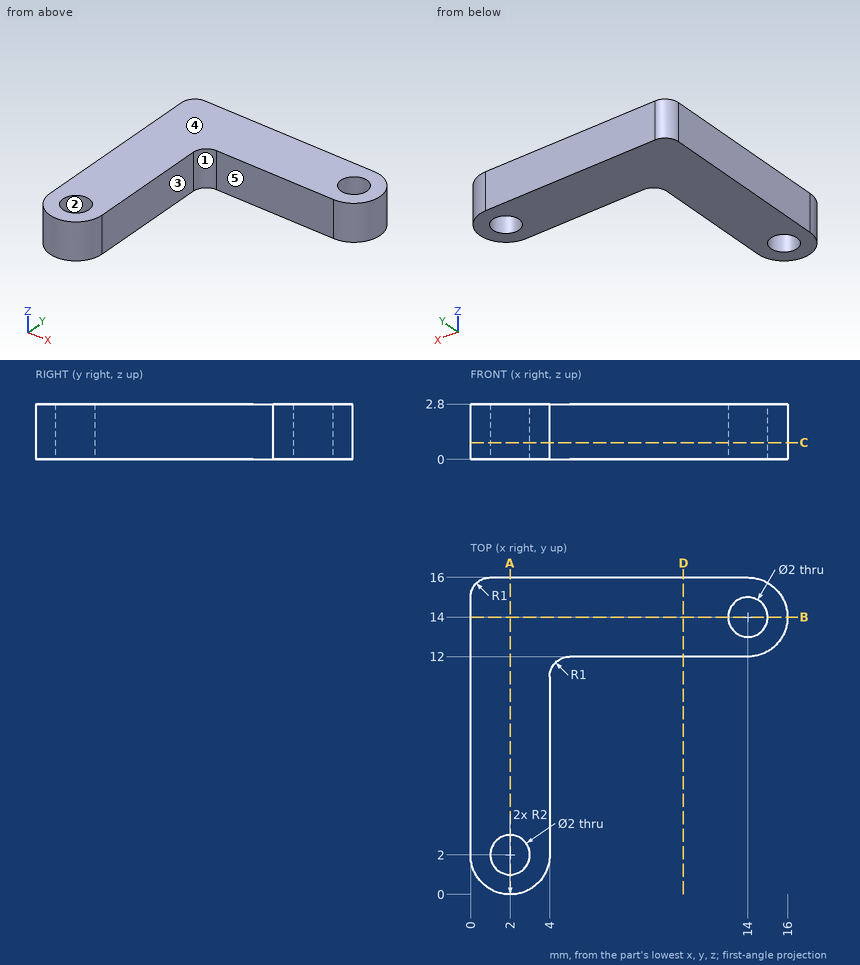
Part print with two shaded views. Sizes in mm from the minimum x, y, z corner. A direction names the side the tool comes from. Round coordinates to 2 decimals unless told otherwise and drop trailing zeros. Order: outer loops, then holes, each group sorted by start corner. A loop starts at its lowest first (then second) coordinate and runs counter-clockwise, first axis right, second up.
(1) 3-axis set-ups, long thin cutter, end or side, ignore diameter. For the marked faces 4 and 5: which of +Z, -Z, +X, -X, +Y, -Y reach the whole face in a straight line?
(2) Band-saw the part on A-A (x = 2). List the corners of the cut face in (y, z), then the cut area to 3 significant figures.
(3) Band-saw the part on C-C (z = 0.85). List the corners of the cut face in (x, y).
(4) Band-saw the part on D-D (x = 10.75). List the corners of the cut face in (y, z).
(5) Pull direction Y, two halves, no side cores. Call the marked faces 1, 2 and 3: released by +Y, released by -Y, zero draft, split by the parting line, or undercut.
(6) Band-saw the part on B-B (y = 14). List the corners of the cut face in (x, z), then the cut area to 3 significant figures.
(7) Pin check, flat tips, straight feed: pin 1 (6 mm diameter, centred on x = 5.5, y = 10, fed in from +Z); pin 2 (1.4 mm diameter, centred on y = 6, z = 1, fed in from +X). Stop position of each tip, or through.
(8) Drill centre lines: line 1 (Y direction, x = 14, z = 2); line 2 (Y direction, x = 6, z = 0.6); line 3 (X direction, y = 7.5, z = 0.1). Where is each one in solid material? Low to high.
Verdict:
1. face 4: +Z, +X, -X, +Y, -Y
1. face 5: +Z, -Z, +X, -Y
2. outline: (0, 0) - (1, 0) - (1, 2.8) - (0, 2.8) - close; (3, 0) - (16, 0) - (16, 2.8) - (3, 2.8) - close
2. area: 39.2 mm2
3. outline: (0, 2) arc R2 ccw to (4, 2) - (4, 11) arc R1 cw to (5, 12) - (14, 12) arc R2 ccw to (14, 16) - (1, 16) arc R1 ccw to (0, 15) - close; hole circle Ø2 at (2, 2); hole circle Ø2 at (14, 14)
4. outline: (12, 0) - (16, 0) - (16, 2.8) - (12, 2.8) - close
5. face 1: released by -Y
5. face 2: undercut
5. face 3: zero draft
6. outline: (0, 0) - (13, 0) - (13, 2.8) - (0, 2.8) - close; (15, 0) - (16, 0) - (16, 2.8) - (15, 2.8) - close
6. area: 39.2 mm2
7. pin 1: stops at z = 2.8
7. pin 2: stops at x = 4
8. line 1: y = 12 to 13, 15 to 16
8. line 2: y = 12 to 16
8. line 3: x = 0 to 4
